```python
from build123d import *

# Parameters (mm, degrees)
EXTRUDE_1_DEPTH     = 50
SKETCH_2_R          = 13
SKETCH_2_R_2        = 2
CUT_EXTRUDE_1_DEPTH = 50
SKETCH_3_R          = 12.5
SKETCH_3_R_2        = 2.5
CUT_EXTRUDE_2_DEPTH = 50


with BuildPart() as part:
    # 草图1 → 凸台-拉伸1 (new body)
    with BuildSketch(Plane(origin=(0, 0, 0), x_dir=(0, 0, -1), z_dir=(1, 0, 0))):
        Polygon((0, 50), (0, 0), (50, 0), (50, 2), (2, 2), (2, 50), align=None)
    extrude(amount=EXTRUDE_1_DEPTH)

    # 草图2 → 切除-拉伸1 (cut)
    with BuildSketch(Plane.XY):
        with Locations((25, 28)):
            Circle(SKETCH_2_R)
        with Locations((7.5, 28)):
            Circle(SKETCH_2_R_2)
        with Locations((25, 45.5)):
            Circle(SKETCH_2_R_2)
        with Locations((25, 10.5)):
            Circle(SKETCH_2_R_2)
        with Locations((42.5, 28)):
            Circle(SKETCH_2_R_2)
    extrude(amount=-CUT_EXTRUDE_1_DEPTH, mode=Mode.SUBTRACT)

    # 草图3 → 切除-拉伸2 (cut)
    with BuildSketch(Plane(origin=(0, 2, 0), x_dir=(1, 0, 0), z_dir=(0, 1, 0))):
        with Locations(Location((25, 26, 0), (0, 0, 270))):
            Circle(SKETCH_3_R)
        with Locations(Location((40, 41, 0), (0, 0, 270))):
            Circle(SKETCH_3_R_2)
        with Locations(Location((40, 11, 0), (0, 0, 270))):
            Circle(SKETCH_3_R_2)
        with Locations(Location((10, 41, 0), (0, 0, 270))):
            Circle(SKETCH_3_R_2)
        with Locations(Location((10, 11, 0), (0, 0, 270))):
            Circle(SKETCH_3_R_2)
    extrude(amount=-CUT_EXTRUDE_2_DEPTH, mode=Mode.SUBTRACT)


solid = part.part
```
Could you check a few things on this model? Use its own coordinates, in mm. A direction names the side the tool comes from. Coordinates: 2 decimals unless noted, no trailing zeros. Loops run counter-clockwise (first coordinate to the right, second up) from the corner with the lowest first, then second, coordinate; pieces in that order, holes last. Notation, with made-up numbers: M 80,25.5 L 114,25.5 A17 cw 114,52.5 Z; hole C 62.25,-34 d9. An arc over 180 degrees is marked long. Put each result on its own line as item: value. Start each with the question number.
(1) Will these pins go through, and if not, where does the flat tip stop? P1, Ø5, axis at x = 7.5, y = 28, coming from the -Z side; P2, Ø8, axis at x = 10, z = -41, coming from the +Y side; P3, Ø1, axis at x = 38.5, y = 10, coming from the +Z side.
(2) Suppose I cut it at D-D on z = -11. Please give me the cut outline in (x, y), then the cut area to 3 significant figures.
(3) I need wall thicknesses on line 1 (Y direction, x = 25, z = -0.65); line 2 (X direction, y = 1.5, z = -11); line 3 (Y direction, x = 3.5, z = -34). Which ranges of each line are inside material? Lowest first, please. Write a range as from..to.
(4) Thinking about a two-plate mould opening in Y: for faces 3 (the face through (30, 0, -14)), 4 (the face through (23.31, 40.89, -0.99)), 5 (the face through (39.04, 1.01, -38.69)), 6 (the face through (25, 50, -1)), which applies, pulls with the +Y half, pulls with the -Y half, needs draft (parallel to the pull), parting line crosses it, or undercut?
(5) Suppose I cut it at B-B on y = 10.5. Please give me the cut outline in (x, z).
(6) Suppose I cut it at C-C on z = -36. Please give me the cut outline in (x, y), then the cut area to 3 significant figures.
(7) Suppose I cut it at A-A on x = 25. Please give me the cut outline in (y, z).
(8) For faces 1 (the face through (9.04, 1.01, -38.69)), 2 (the face through (13.5, 2, -31.7)), which set-ups out of +Z, -Z, +X, -X, +Y, -Y let a thin tool reach every point of the face, with its end or its side?
Solutions:
1. P1: stops at z = -2
1. P2: stops at y = 2
1. P3: stops at z = 0
2. outline: M 0,0 L 7.5,0 L 7.5,2 L 0,2 Z; M 12.5,0 L 37.5,0 L 37.5,2 L 12.5,2 Z; M 42.5,0 L 50,0 L 50,2 L 42.5,2 Z
2. area: 80.0 mm2
3. line 1: y = 0..8.5, 12.5..15, 41..43.5, 47.5..50
3. line 2: x = 0..7.5, 12.5..37.5, 42.5..50
3. line 3: y = 0..2
4. face 3: pulls with the -Y half
4. face 4: undercut
4. face 5: needs draft
4. face 6: pulls with the +Y half
5. outline: M 0,-2 L 23,-2 L 23,0 L 0,0 Z; M 27,-2 L 50,-2 L 50,0 L 27,0 Z
6. outline: M 0,0 L 17.5,0 L 17.5,2 L 0,2 Z; M 32.5,0 L 50,0 L 50,2 L 32.5,2 Z
6. area: 70.0 mm2
7. outline: M 0,-50 L 2,-50 L 2,-38.5 L 0,-38.5 Z; M 0,-13.5 L 2,-13.5 L 2,-2 L 8.5,-2 L 8.5,0 L 0,0 Z; M 12.5,-2 L 15,-2 L 15,0 L 12.5,0 Z; M 41,-2 L 43.5,-2 L 43.5,0 L 41,0 Z; M 47.5,-2 L 50,-2 L 50,0 L 47.5,0 Z
8. face 1: +Y, -Y
8. face 2: -Z, +X, -X, +Y
